Can you work these out from the model? Positions are in its coordinate system, mm. Coordinates: 2 decimals unless noted, no trailing zeros. Loops run counter-clockwise (first coordinate to the right, second up) from the corner with the lowest first, then second, coordinate; pieces in that order, holes last. Notation, with made-up numbers: (86.25, 51.25) -> (95.25, 51.25) arc R19 cw to (95.25, 68.25) -> close; hole circle Ø6 at (31, 89.5). An arc over 180 degrees is marked (long way). Put each result on its own line as item: value. Start each with the question number.
Item 1: Please list where these lines run through material, in increasing order: L1, parallel to X at y = 86, z = 2.3; L2, parallel to Y at x = 594, z = 0.3. Write a range as from..to.
Item 2: If we section it at B-B on x = 574.5: Please give me the cut outline in (y, z), plus the area to 3 significant figures.
Item 3: If we section it at A-A on y = 112: Please give me the cut outline in (x, z).
Item 4: Will these pins go through, and if not, where does the flat tip stop? P1, Ø1.8, axis at x = 492.5, z = 1.5, coming from the -Y side; P2, Ø1.8, axis at x = 494, z = 4, coming from the +Y side; P3, Ø1.8, axis at y = 5, z = 2.5, coming from the +X side.
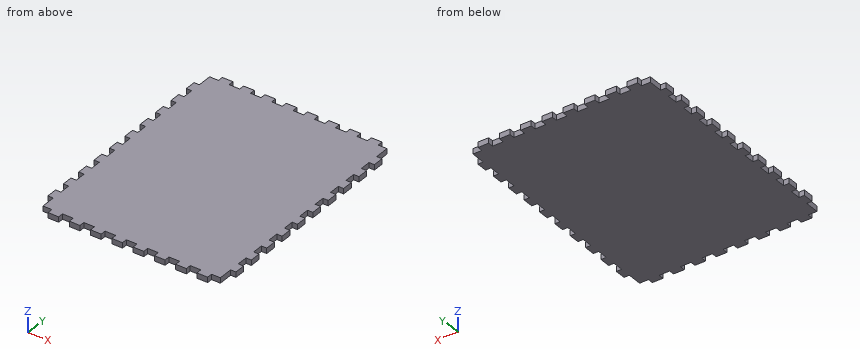
```python
from build123d import *

# Parameters (mm, degrees)
BOSS_EXTRUDE1_DEPTH = 6


with BuildPart() as part:
    # Model → Boss-Extrude1 (new body)
    with BuildSketch(Plane.XY):
        Polygon((496, 269), (496, 253), (490, 253), (490, 241), (496, 241), (496, 229), (490, 229), (490, 217), (496, 217), (496, 205), (490, 205), (490, 193), (496, 193), (496, 181), (490, 181), (490, 169), (496, 169), (496, 157), (490, 157), (490, 145), (496, 145), (496, 133), (490, 133), (490, 121), (496, 121), (496, 109), (490, 109), (490, 97), (496, 97), (496, 85), (490, 85), (490, 73), (496, 73), (496, 61), (490, 61), (490, 49), (496, 49), (496, 37), (490, 37), (490, 25), (496, 25), (496, 13), (496, 9), (506, 9), (506, 3), (518, 3), (518, 9), (530, 9), (530, 3), (542, 3), (542, 9), (554, 9), (554, 3), (566, 3), (566, 9), (578, 9), (578, 3), (590, 3), (590, 9), (602, 9), (602, 3), (614, 3), (614, 9), (626, 9), (626, 3), (638, 3), (638, 9), (650, 9), (650, 3), (662, 3), (662, 9), (674, 9), (674, 3), (686, 3), (686, 9), (696, 9), (696, 25), (702, 25), (702, 37), (696, 37), (696, 49), (702, 49), (702, 61), (696, 61), (696, 73), (702, 73), (702, 85), (696, 85), (696, 97), (702, 97), (702, 109), (696, 109), (696, 121), (702, 121), (702, 133), (696, 133), (696, 145), (702, 145), (702, 157), (696, 157), (696, 169), (702, 169), (702, 181), (696, 181), (696, 193), (702, 193), (702, 205), (696, 205), (696, 217), (702, 217), (702, 229), (696, 229), (696, 241), (702, 241), (702, 253), (696, 253), (696, 265), (696, 269), (686, 269), (686, 275), (674, 275), (674, 269), (662, 269), (662, 275), (650, 275), (650, 269), (638, 269), (638, 275), (626, 275), (626, 269), (614, 269), (614, 275), (602, 275), (602, 269), (590, 269), (590, 275), (578, 275), (578, 269), (566, 269), (566, 275), (554, 275), (554, 269), (542, 269), (542, 275), (530, 275), (530, 269), (518, 269), (518, 275), (506, 275), (506, 269), align=None)
    extrude(amount=BOSS_EXTRUDE1_DEPTH)


solid = part.part
```
Solutions:
1. L1: 496..696
1. L2: 9..269
2. outline: (9, 0) -> (269, 0) -> (269, 6) -> (9, 6) -> close
2. area: 1,560 mm^2
3. outline: (496, 0) -> (696, 0) -> (696, 6) -> (496, 6) -> close
4. P1: y = 25
4. P2: y = 253
4. P3: x = 686
